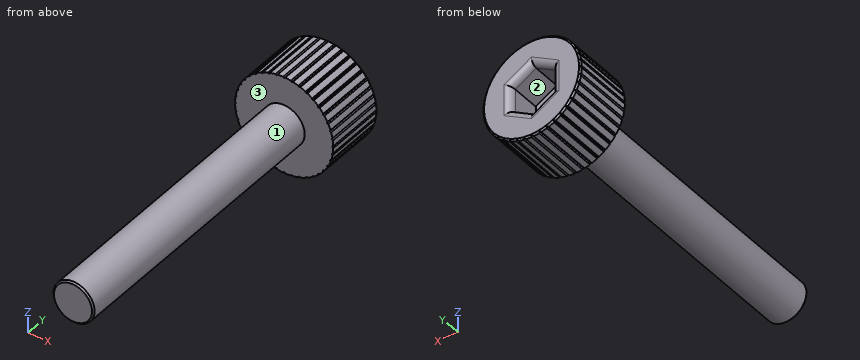
```python
from build123d import *

# Parameters (mm, degrees)
CUT_EXTRUDE1_DEPTH = 4.064
FILLET1_R          = 0.762
CUT_EXTRUDE3_DEPTH = 9.144
CIRPATTERN1_COUNT  = 40


with BuildPart() as part:
    # Sketch1 → Revolve1 (revolve)
    with BuildSketch(Plane.XY):
        Polygon((0, 0), (0, 41.1734), (5.611594878, 41.1734), (5.7912, 40.993794878), (5.7912, 34.036), (2.4257, 34.036), (2.4257, 0.179605122), (2.246094878, 0), align=None)
    revolve(axis=Axis((0, 0, 0), (0, 1, 0)))

    # Sketch2 → Cut-Extrude1 (cut)
    with BuildSketch(Plane(origin=(0, 41.1734, 0), x_dir=(1, 0, 0), z_dir=(0, 1, 0))):
        Polygon((0, -2.8575), (2.474667591, -1.42875), (2.474667591, 1.42875), (0, 2.8575), (-2.474667591, 1.42875), (-2.474667591, -1.42875), align=None)
    extrude(amount=-CUT_EXTRUDE1_DEPTH, mode=Mode.SUBTRACT)

    # Fillet1
    fillet1_edges = [part.edges().sort_by_distance(p)[0] for p in [
        (-1.237333796, 41.1734, 2.143125),
        (1.237333796, 41.1734, 2.143125),
        (2.474667591, 41.1734, 0),
        (1.237333796, 41.1734, -2.143125),
        (-1.237333796, 41.1734, -2.143125),
        (-2.474667591, 41.1734, 0),
    ]]
    fillet(fillet1_edges, radius=FILLET1_R)

    # Sketch3 → Cut-Extrude3 (cut)
    with BuildSketch(Plane(origin=(0, 41.1734, 0), x_dir=(1, 0, 0), z_dir=(0, 1, 0))):
        Polygon((0, 5.6642), (-2.032, 7.6962), (2.032, 7.6962), align=None)
    cut_extrude3 = extrude(amount=-CUT_EXTRUDE3_DEPTH, mode=Mode.SUBTRACT)

    # CirPattern1: Cut-Extrude3 ×40 about axis
    cirpattern1_axis = Axis((0, 0, 0), (0, 1, 0))
    for i in range(1, CIRPATTERN1_COUNT):
        add(cut_extrude3.rotate(cirpattern1_axis, i * 360 / CIRPATTERN1_COUNT), mode=Mode.SUBTRACT)


solid = part.part
```
The listing builds one solid part. Answer for the finished solid, in the listing's coordinates (mm). Face numbers are marked on the shaded views. Coordinates: 2 decimals unless noted, no trailing zeros. Write each loop counter-clockwise with the first axis right and the second up, starting at its lowest first coordinate (ties: lowest second). Pieces come first, ordered by that corner, then holes. Notation, with made-up numbers: (-12, 65.5) - (28, 65.5) arc R23 cw to (28, 99.5) - close; hole circle Ø8 at (-39.5, 50.5). An arc over 180 degrees is marked (long way). Return JSON: item names as keys, results as strings. Group by question number.
Q1. The part is cut by section A-A on y = 28. Write down the section's boundary in (x, z), and give its area (3 significant figures).
Q2. Find the intervals of material crossed by line 1 along Y through (x, z) = (0, 4); line 2 along Z through (x, y) = (1.5, 17); line 3 along X through (y, z) = (34.5, 2.5), in increasing order. Write a range as [from, to].
Q3. For a pull along Z with two mould halves and no side action, classify the marked faces 1, 2 and 3 as +Z half, -Z half, draft (parallel to the pull), parting line (faces both ways), or undercut.
Q4. Flat-ended cylindrical pins translate along their axes: pin 1 Ø5.5 at (x, z) = (-1, -0.5) entering from +Y; pin 2 Ø1 at (x, z) = (0.5, -4) entering from -Y; pin 3 Ø6 at (y, z) = (8, 2) entering from +X; pin 4 Ø1.5 at (x, y) = (-1.5, 4.5) entering from -Z. Find the tip coordinate at first contact, or state that the pin passes through.
Evaluation:
{
 "1": {"outline": "circle Ø4.85 at (0, 0)", "area": "18.5 mm2"},
 "2": {"line 1": "y = [34.04, 41.17]", "line 2": "z = [-1.91, 1.91]", "line 3": "x = [-5.22, 5.22]"},
 "3": {"face 1": "parting line", "face 2": "undercut", "face 3": "draft"},
 "4": {"pin 1": "stops at y = 41.17", "pin 2": "stops at y = 34.04", "pin 3": "stops at x = 2.43", "pin 4": "stops at z = -2.31"}
}
